```python
from build123d import *

# Parameters (mm, degrees)
SKETCH1_R           = 29
BOSS_EXTRUDE1_DEPTH = 90
SKETCH2_R           = 11
BOSS_EXTRUDE2_DEPTH = 28
SKETCH3_R           = 34.6
BOSS_EXTRUDE3_DEPTH = 33
SKETCH4_R           = 2.5
BOSS_EXTRUDE4_DEPTH = 33
SKETCH5_R           = 10
BOSS_EXTRUDE5_DEPTH = 60
SKETCH6_R           = 11
BOSS_EXTRUDE6_DEPTH = 10


with BuildPart() as part:
    # Sketch1 → Boss-Extrude1 (new body)
    with BuildSketch(Plane(origin=(0, 0, 0), x_dir=(1, 0, 0), z_dir=(0, 1, 0))):
        with Locations(Location((0, 0, 0), (0, 0, 90))):
            Circle(SKETCH1_R)
    extrude(amount=BOSS_EXTRUDE1_DEPTH)

    # Sketch2 → Boss-Extrude2 (add)
    with BuildSketch(Plane(origin=(0, 90, 0), x_dir=(1, 0, 0), z_dir=(0, 1, 0))):
        with Locations(Location((0, 0, 0), (0, 0, 270))):
            Circle(SKETCH2_R)
    extrude(amount=BOSS_EXTRUDE2_DEPTH)

    # Sketch3 → Boss-Extrude3 (add)
    with BuildSketch(Plane(origin=(0, 90, 0), x_dir=(1, 0, 0), z_dir=(0, 1, 0))):
        with Locations(Location((0, 0, 0), (0, 0, 270))):
            Circle(SKETCH3_R)
    extrude(amount=-BOSS_EXTRUDE3_DEPTH)

    # Sketch4 → Boss-Extrude4 (add)
    with BuildSketch(Plane(origin=(0, 90, 0), x_dir=(1, 0, 0), z_dir=(0, 1, 0))):
        with Locations((0, 34.6)):
            Circle(SKETCH4_R)
        with Locations((-34.6, 0)):
            Circle(SKETCH4_R)
        with Locations((0, -34.6)):
            Circle(SKETCH4_R)
        with Locations((34.6, 0)):
            Circle(SKETCH4_R)
    extrude(amount=-BOSS_EXTRUDE4_DEPTH)

    # Sketch5 → Boss-Extrude5 (add)
    with BuildSketch(Plane.XY):
        with Locations(Location((-25.665087219, 72.446676229, 0), (0, 0, 207.814921286))):
            Circle(SKETCH5_R)
    extrude(amount=BOSS_EXTRUDE5_DEPTH)

    # Sketch6 → Boss-Extrude6 (add)
    with BuildSketch(Plane.XY.offset(60)):
        with Locations((-25.665087219, 72.446676229)):
            Circle(SKETCH6_R)
    extrude(amount=-BOSS_EXTRUDE6_DEPTH)


solid = part.part
```
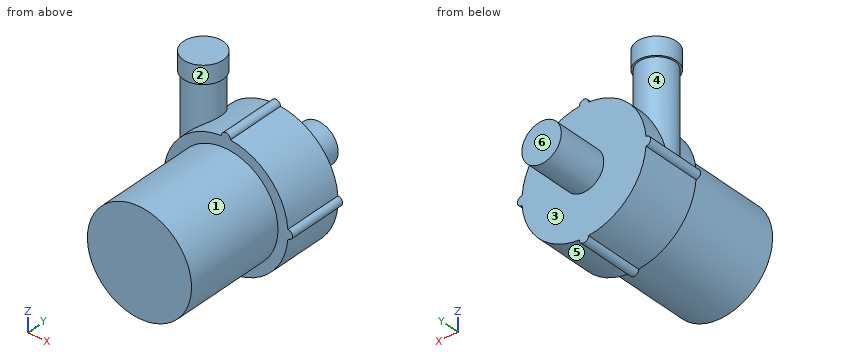
Build history of the part. All positions in model axes, mm. Face numbers are marked on the shaded views. A direction names the side the tool comes from. Give positions to 0.01 mm unless a question says otherwise; leave off trailing zeros. Loops run counter-clockwise (first coordinate to the right, second up) from the corner with the lowest first, then second, coordinate; pieces in that order, holes last.
1) Band-saw the part on B-B on z = 0. List the corners of the cut face in (x, y).
Values follow:
outline: (-37.1, 57) - (-29, 57) - (-29, 0) - (29, 0) - (29, 57) - (37.1, 57) - (37.1, 90) - (11, 90) - (11, 118) - (-11, 118) - (-11, 90) - (-37.1, 90) - close
2) Two-plate mould, pull along Z, no slides. Class the marked faces 4, 5 and 6: released by +Z, released by -Z, zero draft, split by the parting line, or undercut.
Values follow:
face 4: undercut
face 5: released by -Z
face 6: zero draft
3) Band-saw the part on C-C on y = 87. List the corners of the cut face in (x, z).
Values follow:
outline: (-34.51, -2.5) arc R34.6 ccw to (-2.5, -34.51) arc R2.5 ccw (long way) to (2.5, -34.51) arc R34.6 ccw to (34.51, -2.5) arc R2.5 ccw (long way) to (34.51, 2.5) arc R34.6 ccw to (2.5, 34.51) arc R2.5 ccw (long way) to (-2.5, 34.51) arc R34.6 ccw to (-34.51, 2.5) arc R2.5 ccw (long way) to start
4) Band-saw the part on D-D on z = 24.5. List the corners of the cut face in (x, y).
Values follow:
outline: (-24.43, 57) - (-15.52, 57) - (-15.52, 0) - (15.52, 0) - (15.52, 57) - (24.43, 57) - (24.43, 90) - (-24.43, 90) - (-24.43, 82.37) arc R10 ccw (long way) to (-24.43, 62.52) - close
5) Drop flat-ended pins along their axis: P1, Ø5, axis at y = 36, z = 8, coming from the +X side; P2, Ø10, axis at x = 8.5, y = 22, coming from the -Z side; P3, Ø8, axis at x = -0.5, z = 39.5, coming from the +Y side; P4, Ø12, axis at x = 2.5, z = 20, coming from the -Y side. Give the stop position or say it passes through.
Values follow:
P1: stops at x = 28.47
P2: stops at z = -28.79
P3: stops at y = 90
P4: stops at y = 0
6) Band-saw the part on A-A on x = 0. List the corners of the cut face in (y, z).
Values follow:
outline: (0, -29) - (57, -29) - (57, -37.1) - (90, -37.1) - (90, -11) - (118, -11) - (118, 11) - (90, 11) - (90, 37.1) - (57, 37.1) - (57, 29) - (0, 29) - close
7) Probe line 1 along Y through (x, z) = (-4, -28); line 2 along Y through (x, z) = (17.5, -27); line 3 along X through (y, z) = (5, -17). List the from-to ranges inside material, lowest first.
Values follow:
line 1: y = 0 to 90
line 2: y = 57 to 90
line 3: x = -23.49 to 23.49
8) 3-axis set-ups, long thin cutter, end or side, ignore diameter. For the marked faces 1, 2 and 3: which of +Z, -Z, +X, -X, +Y, -Y reach the whole face in a straight line?
Values follow:
face 1: -Y
face 2: +Z
face 3: +Y
